```python
from build123d import *

# Parameters (mm, degrees)
SKETCH_1_W          = 20.4
SKETCH_1_H          = 3
SKETCH_1_R          = 0.6
EXTRUDE_1_DEPTH     = 1.5
FILLET_1_R          = 1.5
CUT_EXTRUDE_START   = 1.5
SKETCH_1_3_R        = 1
CUT_EXTRUDE_1_DEPTH = 0.8


with BuildPart() as part:
    # 草图1 → 凸台-拉伸1 (new body)
    with BuildSketch(Plane(origin=(0, 0, 0), x_dir=(0, 0, -1), z_dir=(1, 0, 0))):
        Rectangle(SKETCH_1_W, SKETCH_1_H)
        Circle(SKETCH_1_R, mode=Mode.SUBTRACT)
        with Locations((-8.7, 0)):
            Circle(SKETCH_1_R, mode=Mode.SUBTRACT)
        with Locations((8.7, 0)):
            Circle(SKETCH_1_R, mode=Mode.SUBTRACT)
    extrude(amount=EXTRUDE_1_DEPTH)

    # 圆角1
    fillet_1_edges = [part.edges().sort_by_distance(p)[0] for p in [
        (0.75, -1.5, -10.2),
        (0.75, 1.5, -10.2),
        (0.75, -1.5, 10.2),
        (0.75, 1.5, 10.2),
    ]]
    fillet(fillet_1_edges, radius=FILLET_1_R - 0.0001)  # a hair under: the kernel refuses the full size

    # 草图1<3> → 切除-拉伸1 (cut)
    with BuildSketch(Plane(origin=(0, 0, 0), x_dir=(0, 0, -1), z_dir=(1, 0, 0)).offset(CUT_EXTRUDE_START)):
        with Locations((-8.7, 0)):
            Circle(SKETCH_1_3_R)
        with Locations((8.7, 0)):
            Circle(SKETCH_1_3_R)
    extrude(amount=-CUT_EXTRUDE_1_DEPTH, mode=Mode.SUBTRACT)


solid = part.part
```
Can you work these out from the model? Positions are in its coordinate system, mm. A direction names the side the tool comes from. Round coordinates to 2 decimals unless told otherwise and drop trailing zeros. Loops run counter-clockwise (first coordinate to the right, second up) from the corner with the lowest first, then second, coordinate; pieces in that order, holes last.
Item 1: Suppose I cut it at B-B, the plane x = 1.25. State how many separate pieces and enclosed holes the cut face has, then the cut area to 3 significant figures.
Item 2: Please list where these lines run through material, in increasing order: L1, parallel to Y at x = 0.5, z = 0; L2, parallel to Z at x = 1.05, y = -0.8; L3, parallel to Z at x = 0.85, y = 0.1.
Item 3: Will this pin go through, and if not, where does the flat tip stop? pin 1 Ø1.4 at (y, z) = (0, -8.7) entering from +X.
Item 4: Suppose I cut it at A-A, the plane z = 0. Write out the boundary of the cut face in (x, y), then the cut area to 3 significant figures.
Item 5: If we mould it in two halves opening along Y, with no side actions, what happens to faces 3 (the cylindrical face through (1.106, 0.3, -9.654)), 4 (the cylindrical face through (0.76, 1.05, 9.77)), 5 (the flat face through (1, -1.5, 0))? For each: +Y half, -Y half, draft (parallel to the pull), parting line (faces both ways), or undercut.
Item 6: Suppose I cut it at C-C, the plane y = -0.3. Write out the boundary of the cut face in (x, z).
Item 7: Which directions (+Z, -Z, +X, -X, +Y, -Y) give clear straight access to the entire face, cutting with the end or side of a thin tool? Please do faces 1 (the cylindrical face through (0.76, 1.07, -9.75)), 2 (the cylindrical face through (1.106, 0.3, 7.746)).
Reported:
1. separate pieces: 1
1. enclosed holes: 3
1. area: 51.9 mm2
2. L1: y = -1.5 to -0.6, 0.6 to 1.5
2. L2: z = -9.97 to -9.3, -8.1 to 8.1, 9.3 to 9.97
2. L3: z = -10.2 to -9.69, -7.71 to -0.59, 0.59 to 7.71, 9.69 to 10.2
3. pin 1: stops at x = 0.7
4. outline: (0, -1.5) - (1.5, -1.5) - (1.5, -0.6) - (0, -0.6) - close; (0, 0.6) - (1.5, 0.6) - (1.5, 1.5) - (0, 1.5) - close
4. area: 2.70 mm2
5. face 3: undercut
5. face 4: +Y half
5. face 5: -Y half
6. outline: (0, -10.17) - (1.5, -10.17) - (1.5, -9.65) - (0.7, -9.65) - (0.7, -9.22) - (0, -9.22) - close; (0, -8.18) - (0.7, -8.18) - (0.7, -7.75) - (1.5, -7.75) - (1.5, -0.52) - (0, -0.52) - close; (0, 0.52) - (1.5, 0.52) - (1.5, 7.75) - (0.7, 7.75) - (0.7, 8.18) - (0, 8.18) - close; (0, 9.22) - (0.7, 9.22) - (0.7, 9.65) - (1.5, 9.65) - (1.5, 10.17) - (0, 10.17) - close
7. face 1: -Z, +X, -X, +Y
7. face 2: +X
